from build123d import *
from build123d.topology import SkipClean

# Parameters (mm, degrees)
SKETCH1_R           = 1.42
BOSS_EXTRUDE1_DEPTH = 5
SKETCH3_R           = 3.25
BOSS_EXTRUDE2_DEPTH = 42


with BuildPart() as part:
    # Sketch1 → Boss-Extrude1 (new body)
    with BuildSketch(Plane(origin=(0, 0, 0), x_dir=(1, 0, 0), z_dir=(0, 1, 0))):
        with BuildLine():
            Line((-8.660254038, -5), (8.660254038, -5))
            ThreePointArc((8.660254038, -5), (0, 10), (-8.660254038, -5))
        make_face()
        with Locations(Location((-5, 0, 0), (0, 0, 270))):
            Circle(SKETCH1_R, mode=Mode.SUBTRACT)
        with Locations(Location((5, 0, 0), (0, 0, 270))):
            Circle(SKETCH1_R, mode=Mode.SUBTRACT)
    extrude(amount=BOSS_EXTRUDE1_DEPTH)

    # Sketch3 → Boss-Extrude2 (add)
    with BuildSketch(Plane(origin=(0, 5, 0), x_dir=(1, 0, 0), z_dir=(0, 1, 0))):
        with Locations(Location((0, 4.734782237, 0), (0, 0, 90))):
            Circle(SKETCH3_R)
    extrude(amount=BOSS_EXTRUDE2_DEPTH)

    # Sketch6 → Revolve1 (revolve)
    with SkipClean():  # the faces are left unmerged after this step: merging them gives an invalid solid
        with BuildSketch(Plane(origin=(0, 47, 0), x_dir=(1, 0, 0), z_dir=(0, 1, 0))):
            with BuildLine():
                ThreePointArc((3.25, 4.734782237), (2.298097039, 7.032879276), (0, 7.984782237))
                Line((0, 7.984782237), (0, 1.484782237))
                ThreePointArc((0, 1.484782237), (2.298097039, 2.436685198), (3.25, 4.734782237))
            make_face()
            with BuildLine():
                Line((0, 1.484782237), (0, 7.984782237))
                ThreePointArc((0, 7.984782237), (-3.25, 4.734782237), (0, 1.484782237))
            make_face()
        revolve(axis=Axis((0, 47, -7.984782237), (0, 0, 1)))


solid = part.part
Model file for the job. Use its own axes, mm. Coordinates: 2 decimals unless noted, no trailing zeros. Write each loop counter-clockwise with the first axis right and the second up, starting at its lowest first coordinate (ties: lowest second). Pieces come first, ordered by that corner, then holes. Notation, with made-up numbers: (29, -9) - (75, -9) arc R8 cw to (75, 6) - close; hole circle Ø6 at (29.25, 7.5). An arc over 180 degrees is marked (long way). Write each question's results on one line, items separated by ' | '. Start each with the question number.
1) Cut at B-B (z = 0). Write the cut outline in (x, y), then the cut area to 3 significant figures.
2) Probe line 1 along X through (y, z) = (1.65, 0); line 2 along Y through (x, z) = (5.75, 3.5); line 3 along Y through (x, z) = (-0.5, -7.5). List the from-to ranges inside material, lowest first. Write a range as from..to.
3) Cut at D-D (x = 0). Write the cut outline in (y, z).
4) Flat gauge pins, fed straight in: P1, Ø10, axis at x = 2.5, y = 43, coming from the -Z side; P2, Ø6, axis at y = 12.5, z = 0, coming from the -X side; P3, Ø8, axis at y = 36.5, z = 1, coming from the +X side. Where does each tip first touch, or does it go through?
5) Cut at A-A (x = -5). Write the cut outline in (y, z).
6) Cut at C-C (z = -4). Write the cut outline in (x, y), then the cut area to 3 significant figures.
7) Mould opens along Z. For faces 1 (the face through (0, 2, 5)), 2 (the face through (6.41, 2.46, -0.18)), 3 (the face through (1.98, 25.71, -2.16)), 4 (the face through (0, 5, -1)) say: pulls with the +Z half, pulls with the -Z half, needs draft (parallel to the pull), parting line crosses it, or undercut.
Returned:
1) outline: (-10, 0) - (-6.42, 0) - (-6.42, 5) - (-10, 5) - close; (-3.58, 0) - (3.58, 0) - (3.58, 5) - (-3.58, 5) - close; (6.42, 0) - (10, 0) - (10, 5) - (6.42, 5) - close | area: 71.6 mm^2
2) line 1: -10..-6.42, -3.58..3.58, 6.42..10 | line 2: 0..5 | line 3: 0..48.63
3) outline: (0, -10) - (5, -10) - (5, -7.98) - (47, -7.98) arc R3.25 ccw to (47, -1.48) - (5, -1.48) - (5, 5) - (0, 5) - close
4) P1: z = -7.98 | P2: x = -2.75 | P3: x = 2.75
5) outline: (0, -8.66) - (5, -8.66) - (5, -1.42) - (0, -1.42) - close; (0, 1.42) - (5, 1.42) - (5, 5) - (0, 5) - close
6) outline: (-9.17, 0) - (9.17, 0) - (9.17, 5) - (3.17, 5) - (3.17, 47) arc R3.17 ccw to (-3.17, 47) - (-3.17, 5) - (-9.17, 5) - close | area: 373 mm^2
7) face 1: pulls with the +Z half | face 2: undercut | face 3: parting line crosses it | face 4: needs draft
